```python
from build123d import *

# Parameters (mm, degrees)
F0_W     = 48
F0_H     = 141
F0_W_2   = 43.2
F0_H_2   = 137.2
F1_DEPTH = 2.4
F2_DEPTH = 22
F3_R     = 10
F4_SCALE = 0.99


with BuildPart() as f1:
    # F0 (on Top) → F1 (new body)
    with BuildSketch(Plane.XY):
        Rectangle(F0_W, F0_H)
        Rectangle(F0_W_2, F0_H_2, mode=Mode.SUBTRACT)
        Rectangle(F0_W_2, F0_H_2)
    extrude(amount=F1_DEPTH)

    # F0 (on Top) → F2 (join)
    with BuildSketch(Plane.XY):
        Rectangle(F0_W, F0_H)
        Rectangle(F0_W_2, F0_H_2, mode=Mode.SUBTRACT)
    extrude(amount=F2_DEPTH)

    # F3
    f3_edges = [f1.edges().sort_by_distance(p)[0] for p in [
        (0, -68.6, 2.4),
        (0, 68.6, 2.4),
    ]]
    fillet(f3_edges, radius=F3_R)


with BuildPart() as f1_1:
    # F4: moved
    add(f1.part.scale(F4_SCALE))


solid = f1_1.part
```
Work out the finished part from the listing and answer in its coordinate system (mm). A direction names the side the tool comes from. Give positions to 0.01 mm unless a question says otherwise; leave off trailing zeros. Order: outer loops, then holes, each group sorted by start corner. A loop starts at its lowest first (then second) coordinate and runs counter-clockwise, first axis right, second up. Notation, with made-up numbers: M -23.75,-38.5 L -17.75,-38.5 A13 ccw -17.75,-15.5 Z; hole C 70,-32 d8. An arc over 180 degrees is marked long. Return JSON: item names as keys, results as strings.
1) A tool of negligible diameter and unlimited length cuts with its end or side. For faces 1 (the flat face through (0, -67.914, 17)), 2 (the flat face through (0, 69.795, 11)), from which of +Z, -Z, +X, -X, +Y, -Y can it reach the whole face along a straight path? Write none if from no direction.
Resolved:
{"face 1": "+Z", "face 2": "+Z, -Z, +X, -X, +Y"}
2) Section B-B, the plane x = -6 is taken. Write down the section's boundary in (y, z) (3 decimals).
Resolved:
{"outline": "M -69.795,0 L 69.795,0 L 69.795,21.78 L 67.914,21.78 L 67.914,12.276 A9.9 cw 58.014,2.376 L -58.014,2.376 A9.9 cw -67.914,12.276 L -67.914,21.78 L -69.795,21.78 Z"}
3) Section A-A, the plane z = 19 is taken. Write down the section's boundary in (x, y) (3 decimals), plus the area to 3 significant figures.
Resolved:
{"outline": "M -23.76,-69.795 L 23.76,-69.795 L 23.76,69.795 L -23.76,69.795 Z; hole M -21.384,-67.914 L 21.384,-67.914 L 21.384,67.914 L -21.384,67.914 Z", "area": "824 mm^2"}
4) Straight lines are drawn through the part: line 1 along X through (y, z) = (-34, 21); line 2 along Y through (x, z) = (-18, 12) (3 decimals); line 3 along Z through (x, y) = (10, 21.5). For each, find the intervals that lie inside material, in ascending order. Write a range as [from, to].
Resolved:
{"line 1": "[-23.76, -21.38], [21.38, 23.76]", "line 2": "[-69.795, -67.91], [67.91, 69.795]", "line 3": "[0, 2.38]"}
5) For a pull along Y with two mould halves and no side action, classify faces 3 (the flat face through (0, 1, 2.376)), 4 (the flat face through (-23.76, -1, 11)), 5 (the flat face through (0, -69.795, 11)) as +Y half, -Y half, draft (parallel to the pull), parting line (faces both ways), or undercut.
Resolved:
{"face 3": "undercut", "face 4": "draft", "face 5": "-Y half"}
6) Section D-D, the plane z = 8.5 is taken. Write down the section's boundary in (x, y) (3 decimals), plus the area to 3 significant figures.
Resolved:
{"outline": "M -23.76,-69.795 L 23.76,-69.795 L 23.76,69.795 L -23.76,69.795 Z; hole M -21.384,-67.166 L 21.384,-67.166 L 21.384,67.166 L -21.384,67.166 Z", "area": "888 mm^2"}
7) Section C-C, the plane y = 43 is taken. Write down the section's boundary in (x, z).
Resolved:
{"outline": "M -23.76,0 L 23.76,0 L 23.76,21.78 L 21.38,21.78 L 21.38,2.38 L -21.38,2.38 L -21.38,21.78 L -23.76,21.78 Z"}
8) This flat-tipped pin is pushed along its axis until it touches: pin 1 (1 mm diameter, centred on x = -8, y = -53.5, fed in from +Z). Where does it stop, or does it pass through?
Resolved:
{"pin 1": "z = 2.38"}
